Geometry check sheet. Reference: the model listing, model coordinates, mm. Round coordinates to 2 decimals unless told otherwise and drop trailing zeros. Loops run counter-clockwise (first coordinate to the right, second up) from the corner with the lowest first, then second, coordinate; pieces in that order, holes last. Notation, with made-up numbers: (43.5, -4.75) -> (102.5, -4.75) arc R15 ccw to (102.5, 8.25) -> close; hole circle Ø9 at (-9.75, 69). An arc over 180 degrees is marked (long way). Use one line per item in the form item = value.
from build123d import *

# Parameters (mm, degrees)
SKETCH1_W           = 110
SKETCH1_H           = 15
BOSS_EXTRUDE1_DEPTH = 3
CUT_EXTRUDE1_REACH  = 57.59
SKETCH2_R           = 3
FILLET1_R           = 5


with BuildPart() as part:
    # Sketch1 → Boss-Extrude1 (new body)
    with BuildSketch(Plane(origin=(0, 0, 0), x_dir=(1, 0, 0), z_dir=(0, 1, 0))):
        Rectangle(SKETCH1_W, SKETCH1_H)
    extrude(amount=BOSS_EXTRUDE1_DEPTH)

    # Sketch2 → Cut-Extrude1 (cut, up to next)
    with BuildSketch(Plane(origin=(0, 3, 0), x_dir=(1, 0, 0), z_dir=(0, 1, 0)), mode=Mode.PRIVATE) as cut_extrude1_sk1:
        with Locations(Location((-49, 0, 0), (0, 0, 270))):
            Circle(SKETCH2_R)
    cut_extrude1_tool1 = extrude(cut_extrude1_sk1.sketch, amount=-CUT_EXTRUDE1_REACH, mode=Mode.PRIVATE) & part.part
    # Sketch2 → Cut-Extrude1 (cut, up to next)
    with BuildSketch(Plane(origin=(0, 3, 0), x_dir=(1, 0, 0), z_dir=(0, 1, 0)), mode=Mode.PRIVATE) as cut_extrude1_sk2:
        with Locations(Location((-39, 0, 0), (0, 0, 270))):
            Circle(SKETCH2_R)
    cut_extrude1_tool2 = extrude(cut_extrude1_sk2.sketch, amount=-CUT_EXTRUDE1_REACH, mode=Mode.PRIVATE) & part.part
    cut_extrude1_1 = cut_extrude1_tool1.solids().sort_by_distance((-49, 3, 0))[0]
    add(cut_extrude1_1, mode=Mode.SUBTRACT)
    cut_extrude1_2 = cut_extrude1_tool2.solids().sort_by_distance((-39, 3, 0))[0]
    add(cut_extrude1_2, mode=Mode.SUBTRACT)
    cut_extrude1 = cut_extrude1_1 + cut_extrude1_2  # Cut-Extrude1 as one shape, for the pattern or mirror that repeats it

    # Mirror1: Cut-Extrude1 across plane
    add(cut_extrude1.mirror(Plane(origin=(0, 0, 0), x_dir=(0, 0, 1), z_dir=(1, 0, 0))), mode=Mode.SUBTRACT)

    # Fillet1
    fillet1_edges = [part.edges().sort_by_distance(p)[0] for p in [
        (-55, 1.5, -7.5),
        (55, 1.5, -7.5),
        (55, 1.5, 7.5),
        (-55, 1.5, 7.5),
    ]]
    fillet(fillet1_edges, radius=FILLET1_R)


solid = part.part
1. Mould release check, pull along Z, two halves, no side actions. Record for faces 1 (the flat face through (-55, 1, 0)), 2 (the cylindrical face through (46, 2, 0)), 3 (the flat face through (-1, 1, -7.5)): released by +Z, released by -Z, zero draft, split by the parting line, or undercut.
Return value:
face_1 = zero draft
face_2 = undercut
face_3 = released by -Z
2. Section check A-A (x = -39). Record the boundary of the cut face in (y, z).
Return value:
outline = (0, -7.5) -> (3, -7.5) -> (3, -3) -> (0, -3) -> close; (0, 3) -> (3, 3) -> (3, 7.5) -> (0, 7.5) -> close
3. Gauge pin test, flat end, axial feed: pin 1 (3.5 mm diameter, centred on x = -49, z = 0, fed in from -Y). Record the tip position at first contact, or that the pin passes through.
Return value:
pin_1 = through
4. Section check D-D (z = -6). Record the boundary of the cut face in (x, y), then the cut area to 3 significant figures.
Return value:
outline = (-53.57, 0) -> (53.57, 0) -> (53.57, 3) -> (-53.57, 3) -> close
area = 321 mm2
5. Section check B-B (z = 0). Record the boundary of the cut face in (x, y), then the cut area to 3 significant figures.
Return value:
outline = (-55, 0) -> (-52, 0) -> (-52, 3) -> (-55, 3) -> close; (-46, 0) -> (-42, 0) -> (-42, 3) -> (-46, 3) -> close; (-36, 0) -> (36, 0) -> (36, 3) -> (-36, 3) -> close; (42, 0) -> (46, 0) -> (46, 3) -> (42, 3) -> close; (52, 0) -> (55, 0) -> (55, 3) -> (52, 3) -> close
area = 258 mm2
6. Section check C-C (y = 0.7). Record the boundary of the cut face in (x, z).
Return value:
outline = (-55, -2.5) arc R5 ccw to (-50, -7.5) -> (50, -7.5) arc R5 ccw to (55, -2.5) -> (55, 2.5) arc R5 ccw to (50, 7.5) -> (-50, 7.5) arc R5 ccw to (-55, 2.5) -> close; hole circle Ø6 at (-49, 0); hole circle Ø6 at (-39, 0); hole circle Ø6 at (39, 0); hole circle Ø6 at (49, 0)
7. Material ranges on line 1 along X through (y, z) = (1.85, 0); line 2 along X through (y, z) = (0.5, 1); line 3 along Z through (x, y) = (49, 1.8), recorded low to high.
Return value:
line_1 = -55 to -52, -46 to -42, -36 to 36, 42 to 46, 52 to 55
line_2 = -55 to -51.83, -46.17 to -41.83, -36.17 to 36.17, 41.83 to 46.17, 51.83 to 55
line_3 = -7.5 to -3, 3 to 7.5
